```python
from build123d import *

# Parameters (mm, degrees)
F0_W      = 27
F0_H      = 31
F1_DEPTH  = 1.5
F3_DEPTH  = 27
F4_W      = 27
F4_H      = 19
F5_DEPTH  = 2.5
F6_R      = 2
F7_W      = 12
F7_H      = 4.15
F8_DEPTH  = 25
F9_R      = 1.25
F10_DEPTH = 2
F11_R     = 0.6


with BuildPart() as f1:
    # F0 (on Top) → F1 (new body)
    with BuildSketch(Plane.XY):
        with Locations((-3.0333630769, 4.2747315317)):
            Rectangle(F0_W, F0_H)
    extrude(amount=F1_DEPTH)

    # F2 (on face) → F3 (join)
    with BuildSketch(Plane(origin=(-16.5333630769, 0, 0), x_dir=(0, -1, 0), z_dir=(-1, 0, 0))):
        Polygon((-19.7747315317, 1.5), (11.2252684683, 1.5), (-12.816344435, 14.434096374), align=None)
    extrude(amount=-F3_DEPTH)

    # F4 (on face) → F5 (cut)
    with BuildSketch(Plane(origin=(0, -3.1455131558, 5.846810437), x_dir=(1, 0, 0), z_dir=(0, -0.473776424, 0.8806451613))):
        with Locations((-3.0333630769, 4.4751862752)):
            Rectangle(F4_W, F4_H)
    extrude(amount=-F5_DEPTH, mode=Mode.SUBTRACT)

    # F6
    f6_edges = [f1.edges().sort_by_distance(p)[0] for p in [
        (-3.033363, 10.346108, 10.266311),
        (-3.033363, -6.38615, 1.264559),
    ]]
    fillet(f6_edges, radius=F6_R)

    # F7 (on face) → F8 (cut)
    with BuildSketch(Plane(origin=(0, -3.1455131558, 5.846810437), x_dir=(1, 0, 0), z_dir=(0, -0.473776424, 0.8806451613))):
        with Locations((-3.0333630769, 16.0501862752)):
            Rectangle(F7_W, F7_H)
    extrude(amount=-F8_DEPTH, mode=Mode.SUBTRACT)

    # F9 (on face) → F10 (join)
    with BuildSketch(Plane(origin=(0, -3.1455131558, 5.846810437), x_dir=(1, 0, 0), z_dir=(0, -0.473776424, 0.8806451613))):
        with Locations((-13.2333630769, 16.0751862752)):
            Circle(F9_R)
        with Locations((7.1666369231, 16.0751862752)):
            Circle(F9_R)
        with Locations((-13.2333630769, -7.1248137248)):
            Circle(F9_R)
        with Locations((7.1666369231, -7.1248137248)):
            Circle(F9_R)
    extrude(amount=F10_DEPTH)

    # F11
    f11_edges = [f1.edges().sort_by_distance(p)[0] for p in [
        (-14.483363, -10.367499, 4.232532),
        (5.916637, -10.367499, 4.232532),
        (-14.483363, 10.063469, 15.224145),
        (5.916637, 10.063469, 15.224145),
    ]]
    fillet(f11_edges, radius=F11_R)


solid = f1.part
```
Here's how the part is built. I have some questions about the finished solid (model axes, mm). A direction names the side the tool comes from. Coordinates: 2 decimals unless noted, no trailing zeros. Loops run counter-clockwise (first coordinate to the right, second up) from the corner with the lowest first, then second, coordinate; pieces in that order, holes last. Notation, with made-up numbers: (-30.5, 71.5) - (24.5, 71.5) arc R18 cw to (24.5, 85.5) - close; hole circle Ø11 at (78, 55.5). An arc over 180 degrees is marked (long way). Answer as CSV lines item,"result".
Q1. For pin 1 (8 mm diameter, centred on x = -11.5, z = 13.5, fed in from +Y); pin 2 (1 mm diameter, centred on x = 1.5, y = 16, fed in from +Z); pin 3 (3 mm diameter, centred on x = 0, z = 4, fed in from +Y), each with a flat end and sliding along its axis, tell me the tip position at first contact or that it passes through.
Response:
pin 1,"y = 15.47"
pin 2,"z = 0.69"
pin 3,"y = 14.52"
Q2. If we section it at A-A, the plane x = -9.5: Write out the boundary of the cut face in (y, z).
Response:
outline,"(-11.23, 0) - (19.77, 0) - (19.77, 1.5) - (12.82, 14.43) - (9.16, 12.47) - (9.4, 12.03) arc R2 cw to (8.58, 9.32) - (-4.62, 2.21) arc R2 cw to (-7.33, 3.03) - (-7.57, 3.47) - (-11.23, 1.5) - close"
Q3. If we section it at D-D, the plane y = 0.5: Write out the boundary of the cut face in (x, z), and give its area (3 significant figures).
Response:
outline,"(-16.53, 0) - (10.47, 0) - (10.47, 4.97) - (-16.53, 4.97) - close"
area,"134 mm2"
Q4. We'd pull the mould along Z, two halves only. Please class faces 1 (the face through (-3, -11.225, 1)), 2 (the face through (-13.242, -10.359, 4.237)), 3 (the face through (-2.84, 9.56, 10.53)), 4 (the face through (-3, 4, 0)): pulls with the +Z half, pulls with the -Z half, needs draft (parallel to the pull), parting line crosses it, or undercut.
Response:
face 1,"needs draft"
face 2,"pulls with the +Z half"
face 3,"undercut"
face 4,"pulls with the -Z half"
Q5. If I drill on L1, parallel to X at y = 11, z = 10; L2, parallel to X at y = 10.5, z = 14.75; L3, parallel to Z at x = 2.25, y = 5, over which ranges is the centre line in solid material (lowest first)? Write a range as [from, to].
Response:
L1,"[-16.53, -9.03], [2.97, 10.47]"
L2,"[-14.47, -11.99], [5.93, 8.41]"
L3,"[0, 7.39]"
Q6. If we section it at C-C, the plane y = 13.5: Write out the boundary of the cut face in (x, z).
Response:
outline,"(-16.53, 0) - (10.47, 0) - (10.47, 13.16) - (2.97, 13.16) - (2.97, 4.4) - (-9.03, 4.4) - (-9.03, 13.16) - (-16.53, 13.16) - close"
Q7. For faces 5 (the face through (-9.033, 15, 6)), 6 (the face through (8.36, 11.01, 14.25)), 7 (the face through (-3.222, 2.072, 5.815)), which set-ups out of +Z, -Z, +X, -X, +Y, -Y let a thin tool reach every point of the face, with its end or its side?
Response:
face 5,"+Z, +Y"
face 6,"none"
face 7,"+Z, +X, -X"
Q8. If we section it at B-B, the plane z = 6.5: Write out the boundary of the cut face in (x, y).
Response:
outline,"(-16.53, 3.35) - (10.47, 3.35) - (10.47, 17.08) - (2.97, 17.08) - (2.97, 12.37) - (-9.03, 12.37) - (-9.03, 17.08) - (-16.53, 17.08) - close"
